```python
from build123d import *

# Parameters (mm, degrees)
F0_W     = 60
F0_H     = 60
F0_R     = 3.25
F0_R_2   = 20.25
F1_DEPTH = 5
F2_R     = 5
F3_R     = 19.5
F4_DEPTH = 5
F5_R     = 25
F5_R_2   = 17.5
F6_DEPTH = 20


with BuildPart() as f1:
    # F0 (on Top) → F1 (new body)
    with BuildSketch(Plane.XY):
        Rectangle(F0_W, F0_H)
        with Locations((-20.75, -20.75)):
            Circle(F0_R, mode=Mode.SUBTRACT)
        with Locations((20.75, -20.75)):
            Circle(F0_R, mode=Mode.SUBTRACT)
        with Locations((-20.75, 20.75)):
            Circle(F0_R, mode=Mode.SUBTRACT)
        Circle(F0_R_2, mode=Mode.SUBTRACT)
        with Locations((20.75, 20.75)):
            Circle(F0_R, mode=Mode.SUBTRACT)
    extrude(amount=F1_DEPTH)

    # F2
    f2_edges = [f1.edges().sort_by_distance(p)[0] for p in [
        (-30, -30, 2.5),
        (30, -30, 2.5),
        (30, 30, 2.5),
        (-30, 30, 2.5),
    ]]
    fillet(f2_edges, radius=F2_R)

    # F3 (on face) → F4 (cut)
    with BuildSketch(Plane.XY.offset(5)):
        Circle(F3_R)
    extrude(amount=-F4_DEPTH, mode=Mode.SUBTRACT)

    # F5 (on face) → F6 (join)
    with BuildSketch(Plane(origin=(0, 0, 0), x_dir=(1, 0, 0), z_dir=(0, 0, -1))):
        Circle(F5_R)
        Circle(F5_R_2, mode=Mode.SUBTRACT)
    extrude(amount=F6_DEPTH)


solid = f1.part
```
CAD build for the part. Positions are in the model's coordinates, mm. A direction names the side the tool comes from. Round coordinates to 2 decimals unless told otherwise and drop trailing zeros. Order: outer loops, then holes, each group sorted by start corner. A loop starts at its lowest first (then second) coordinate and runs counter-clockwise, first axis right, second up.
Item 1: Saw through at C-C on z = 1.25. Write the cut outline in (x, y), then the cut area to 3 significant figures.
Item 2: Tool access for faces 1 (the face through (23.846, -7.509, -9.86)), 2 (the face through (-17, 6, 0)), 3 (the face through (17.503, -20.607, 2.465)): list every direction of +Z, -Z, +X, -X, +Y, -Y with a clear straight run to the whole face (end or side of a thin tool).
Item 3: Saw through at A-A on y = 0. Write the cut outline in (x, z), then the cut area to 4 significant figures.
Item 4: Probe line 1 along Y through (x, z) = (20.75, 4.05); line 2 along Y through (x, z) = (0, -7.5); line 3 along Y through (x, z) = (0, 3.6). List the from-to ranges inside material, lowest first.
Item 5: Pin check, flat tips, straight feed: pin 1 (2 mm diameter, centred on x = -13, z = -11, fed in from +Y); pin 2 (8.5 mm diameter, centred on x = 20.75, y = 20.75, fed in from -Z); pin 3 (6 mm diameter, centred on y = 19.5, z = -12, fed in from -X). Stop position of each tip, or through.
Item 6: Saw through at D-D on z = -10.5. Write the cut outline in (x, y).
Reported:
1. outline: (-30, -25) arc R5 ccw to (-25, -30) - (25, -30) arc R5 ccw to (30, -25) - (30, 25) arc R5 ccw to (25, 30) - (-25, 30) arc R5 ccw to (-30, 25) - close; hole circle Ø6.5 at (-20.75, -20.75); hole circle Ø6.5 at (-20.75, 20.75); hole circle Ø40.5 at (0, 0); hole circle Ø6.5 at (20.75, -20.75); hole circle Ø6.5 at (20.75, 20.75)
1. area: 2,160 mm2
2. face 1: -Z
2. face 2: +Z
2. face 3: +Z, -Z
3. outline: (-30, 0) - (-25, 0) - (-25, -20) - (-17.5, -20) - (-17.5, 0) - (-20.25, 0) - (-20.25, 5) - (-30, 5) - close; (17.5, -20) - (25, -20) - (25, 0) - (30, 0) - (30, 5) - (20.25, 5) - (20.25, 0) - (17.5, 0) - close
3. area: 397.5 mm2
4. line 1: y = -30 to -24, -17.5 to 17.5, 24 to 30
4. line 2: y = -25 to -17.5, 17.5 to 25
4. line 3: y = -30 to -20.25, 20.25 to 30
5. pin 1: stops at y = 21.93
5. pin 2: stops at z = 0
5. pin 3: stops at x = -18.78
6. outline: circle Ø50 at (0, 0); hole circle Ø35 at (0, 0)
